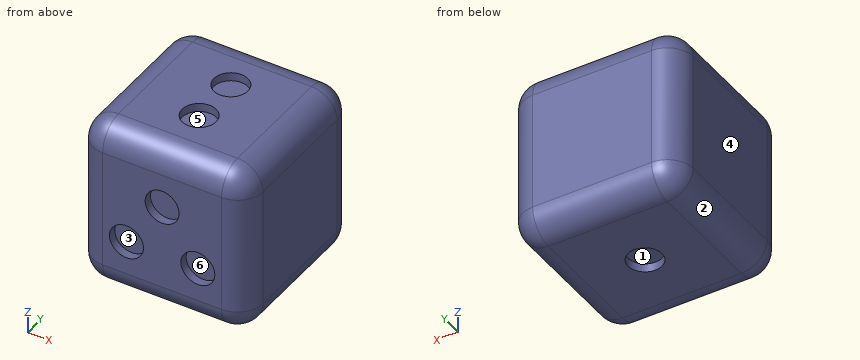
from build123d import *

# Parameters (mm, degrees)
F0_W      = 100
F0_H      = 100
F1_DEPTH  = 100
F2_F1_R   = 15
F2_F2_R   = 15
F2_F3_R   = 15
F2_F4_R   = 15
F2_F5_R   = 15
F4_R      = 10
F5_DEPTH  = 5
F7_R      = 10
F8_DEPTH  = 5
F9_R      = 10
F10_DEPTH = 5


# Not quite as in the source:
# - a feature of the source that left no trace in its solid (it failed there, or was rolled back) is left out


with BuildPart() as f1:
    # F0 (on Top) → F1 (new body)
    with BuildSketch(Plane.XY):
        Rectangle(F0_W, F0_H)
    extrude(amount=F1_DEPTH)

    # F2: fillet of radius 15 on 7 edges, made by hand

    # F2_f1
    f2_f1_edges = [f1.edges().sort_by_distance(p)[0] for p in [
        (50, 50, 50),
    ]]
    fillet(f2_f1_edges, radius=F2_F1_R)

    # F2_f2
    f2_f2_edges = [f1.edges().sort_by_distance(p)[0] for p in [
        (-50, 50, 50),
    ]]
    fillet(f2_f2_edges, radius=F2_F2_R)

    # F2_f3
    f2_f3_edges = [f1.edges().sort_by_distance(p)[0] for p in [
        (0, 50, 100),
    ]]
    fillet(f2_f3_edges, radius=F2_F3_R)

    # F2_f4
    f2_f4_edges = [f1.edges().sort_by_distance(p)[0] for p in [
        (-50, -50, 42.5),
    ]]
    fillet(f2_f4_edges, radius=F2_F4_R)

    # F2_f5
    f2_f5_edges = [f1.edges().sort_by_distance(p)[0] for p in [
        (-50, 0, 0),
    ]]
    fillet(f2_f5_edges, radius=F2_F5_R)

    # F4 (on Top) → F5 (cut)
    with BuildSketch(Plane.XY):
        Circle(F4_R)
    extrude(amount=F5_DEPTH, mode=Mode.SUBTRACT)

    # F7 (on face) → F8 (cut)
    with BuildSketch(Plane.XY.offset(100)):
        with Locations((0, -15)):
            Circle(F7_R)
        with Locations((0, 15)):
            Circle(F7_R)
    extrude(amount=-F8_DEPTH, mode=Mode.SUBTRACT)

    # F9 (on face) → F10 (cut)
    with BuildSketch(Plane.XZ.offset(50)):
        with Locations((0, 65)):
            Circle(F9_R)
        with Locations((-21, 35)):
            Circle(F9_R)
        with Locations((21, 35)):
            Circle(F9_R)
    extrude(amount=-F10_DEPTH, mode=Mode.SUBTRACT)


solid = f1.part
Read the model definition and answer for the solid it produces. Units are mm, in the model's axes. Face numbers are marked on the shaded views. A direction names the side the tool comes from. Coordinates: 2 decimals unless noted, no trailing zeros. Loops run counter-clockwise (first coordinate to the right, second up) from the corner with the lowest first, then second, coordinate; pieces in that order, holes last.
Q1. Each of these flat-tipped pins is pushed along its axis until it touches: pin 1 Ø6 at (x, z) = (-2.5, 60.5) entering from -Y; pin 2 Ø16 at (x, y) = (-1, -15) entering from +Z; pin 3 Ø6 at (x, y) = (2.5, -2) entering from -Z. Where does it stop, or does it pass through?
Q2. The part is cut by section C-C on x = -21. Write down the section's boundary in (y, z), and give its area (3 significant figures).
Q3. The mould has two halves that part along Y. Classify the marked faces 4, 5 and 6: +Y half, -Y half, draft (parallel to the pull), parting line (faces both ways), or undercut.
Q4. The part is cut by section A-A on z = 35. Write down the section's boundary in (x, y), and give its area (3 significant figures).
Q5. Which of the six approach directions +Z, -Z, +X, -X, +Y, -Y give full straight-line access (tool end or side, diameter ignored) to the marked faces 1, 2 and 3?
Q6. The part is cut by section D-D on x = 0. Write down the section's boundary in (y, z), and give its area (3 significant figures).
Q7. Consider probe 1 along Y at (x, z) = (0, 97); probe 2 along Y at (x, z) = (-8.5, 69); probe 3 along Z at (x, y) = (4, -2). Determine where each line is inside the solid, lowest interval first.
Q8. The part is cut by section B-B on y = -15. Write down the section's boundary in (x, z).
Results below:
1. pin 1: stops at y = -45
1. pin 2: stops at z = 95
1. pin 3: stops at z = 5
2. outline: (-50, 15) arc R15 ccw to (-35, 0) - (35, 0) arc R15 ccw to (50, 15) - (50, 85) arc R15 ccw to (35, 100) - (-35, 100) arc R15 ccw to (-50, 85) - (-50, 45) - (-45, 45) - (-45, 25) - (-50, 25) - close
2. area: 9,710 mm2
3. face 4: draft
3. face 5: undercut
3. face 6: -Y half
4. outline: (-50, -35) arc R15 ccw to (-35, -50) - (-31, -50) - (-31, -45) - (-11, -45) - (-11, -50) - (11, -50) - (11, -45) - (31, -45) - (31, -50) - (35, -50) arc R15 ccw to (50, -35) - (50, 35) arc R15 ccw to (35, 50) - (-35, 50) arc R15 ccw to (-50, 35) - close
4. area: 9,610 mm2
5. face 1: -Z
5. face 2: -Z, -X, +Y, -Y
5. face 3: -Y
6. outline: (-50, 15) arc R15 ccw to (-35, 0) - (-10, 0) - (-10, 5) - (10, 5) - (10, 0) - (35, 0) arc R15 ccw to (50, 15) - (50, 85) arc R15 ccw to (35, 100) - (25, 100) - (25, 95) - (5, 95) - (5, 100) - (-5, 100) - (-5, 95) - (-25, 95) - (-25, 100) - (-35, 100) arc R15 ccw to (-50, 85) - (-50, 75) - (-45, 75) - (-45, 55) - (-50, 55) - close
6. area: 9,410 mm2
7. probe 1: y = -44 to -25, -5 to 5, 25 to 44
7. probe 2: y = -45 to 50
7. probe 3: z = 5 to 100
8. outline: (-50, 15) arc R15 ccw to (-35, 0) - (35, 0) arc R15 ccw to (50, 15) - (50, 85) arc R15 ccw to (35, 100) - (10, 100) - (10, 95) - (-10, 95) - (-10, 100) - (-35, 100) arc R15 ccw to (-50, 85) - close
